```python
from build123d import *

# Parameters (mm, degrees)
SKETCH1_W               = 269.4
SKETCH1_H               = 265.6
BOSS_EXTRUDE1_DEPTH     = 3.175
CUT_EXTRUDE3_DEPTH      = 190.262390612
BOSS_EXTRUDE3_DEPTH     = 6.35
F_1_4_CLEARANCE_HOLE1_D = 6.7564
MIRROR2_COPY_1_DEPTH    = 6.35
MIRROR2_COPY_2_D        = 6.7564
CUT_EXTRUDE2_REACH      = 191.262
SKETCH15_W              = 0.944
SKETCH15_H              = 50.8
LPATTERN1_COUNT         = 8
LPATTERN1_PITCH         = 10
MIRROR3_COPY_1_REACH    = 191.262
MIRROR3_COPY_1_SKETCH_W = 0.944
MIRROR3_COPY_1_SKETCH_H = 50.8
MIRROR3_COPY_2_REACH    = 191.262
MIRROR3_COPY_2_SKETCH_W = 0.944
MIRROR3_COPY_2_SKETCH_H = 50.8
MIRROR3_COPY_3_REACH    = 191.262
MIRROR3_COPY_3_SKETCH_W = 0.944
MIRROR3_COPY_3_SKETCH_H = 50.8
MIRROR3_COPY_4_REACH    = 191.262
MIRROR3_COPY_4_SKETCH_W = 0.944
MIRROR3_COPY_4_SKETCH_H = 50.8
MIRROR3_COPY_5_REACH    = 191.262
MIRROR3_COPY_5_SKETCH_W = 0.944
MIRROR3_COPY_5_SKETCH_H = 50.8
MIRROR3_COPY_6_REACH    = 191.262
MIRROR3_COPY_6_SKETCH_W = 0.944
MIRROR3_COPY_6_SKETCH_H = 50.8
MIRROR3_COPY_7_REACH    = 191.262
MIRROR3_COPY_7_SKETCH_W = 0.944
MIRROR3_COPY_7_SKETCH_H = 50.8


with BuildPart() as part:
    # Sketch1 → Boss-Extrude1 (new, symmetric)
    with BuildSketch(Plane(origin=(0, 0, 0), x_dir=(1, 0, 0), z_dir=(0, 1, 0))):
        Rectangle(SKETCH1_W, SKETCH1_H)
    extrude(amount=BOSS_EXTRUDE1_DEPTH, both=True)

    # Sketch16 → Cut-Extrude3 (cut, through all)
    with BuildSketch(Plane(origin=(0, 3.175, 0), x_dir=(1, 0, 0), z_dir=(0, 1, 0))):
        Polygon((-134.7, 132.8), (-134.7, 91.434816919), (-99.990490133, 132.8), align=None)
        Polygon((99.990490133, 132.8), (134.7, 132.8), (134.7, 91.434816919), align=None)
        Polygon((134.7, -132.8), (134.7, -91.434816919), (99.990490133, -132.8), align=None)
        Polygon((-99.990490133, -132.8), (-134.7, -132.8), (-134.7, -91.434816919), align=None)
    extrude(amount=-CUT_EXTRUDE3_DEPTH, mode=Mode.SUBTRACT)

    # Sketch7 → Boss-Extrude3 (add)
    with BuildSketch(Plane(origin=(0, -3.175, 0), x_dir=(1, 0, 0), z_dir=(0, 1, 0))):
        Polygon((126.560486405, 125.832227239), (132.451914797, 118.811096288), (126.182387654, 101.585712032), (108.508102479, 122.649104887), align=None)
    boss_extrude3 = extrude(amount=BOSS_EXTRUDE3_DEPTH)

    # 1/4 Clearance Hole1 (through all)
    with Locations(Plane.XZ.offset(3.175)):
        with Locations((123.415994069, -117.211371709), (126.7498, -40), (0, -124.8498)):
            f_1_4_clearance_hole1 = Hole(F_1_4_CLEARANCE_HOLE1_D / 2)

    # Mirror1: Boss-Extrude3, 1/4 Clearance Hole1 across plane
    add(boss_extrude3.mirror(Plane.XY))
    add(f_1_4_clearance_hole1.mirror(Plane.XY), mode=Mode.SUBTRACT)

    # Mirror2: Boss-Extrude3, 1/4 Clearance Hole1 across plane
    add(boss_extrude3.mirror(Plane(origin=(0, 0, 0), x_dir=(0, 0, 1), z_dir=(1, 0, 0))))
    add(f_1_4_clearance_hole1.mirror(Plane(origin=(0, 0, 0), x_dir=(0, 0, 1), z_dir=(1, 0, 0))), mode=Mode.SUBTRACT)

    # Mirror2 copy 1 sketch → Mirror2 copy 1 (add)
    with BuildSketch(Plane(origin=(0, -3.175, 0), x_dir=(-1, 0, 0), z_dir=(0, 1, 0))):
        Polygon((126.560486405, 125.832227239), (132.451914797, 118.811096288), (126.182387654, 101.585712032), (108.508102479, 122.649104887), align=None)
    extrude(amount=MIRROR2_COPY_1_DEPTH)

    # Mirror2 copy 2 (through all)
    with Locations(Plane(origin=(0, -3.175, 0), x_dir=(-1, 0, 0), z_dir=(0, -1, 0))):
        with Locations((123.415994069, -117.211371709), (126.7498, -40), (0, -124.8498)):
            Hole(MIRROR2_COPY_2_D / 2)

    # Sketch15 → Cut-Extrude2 (cut, up to next)
    with BuildSketch(Plane(origin=(0, 3.175, 0), x_dir=(1, 0, 0), z_dir=(0, 1, 0)), mode=Mode.PRIVATE) as cut_extrude2_sk1:
        with Locations((-88.499, -97.4)):
            Rectangle(SKETCH15_W, SKETCH15_H)
    cut_extrude2_tool1 = extrude(cut_extrude2_sk1.sketch, amount=-CUT_EXTRUDE2_REACH, mode=Mode.PRIVATE) & part.part
    cut_extrude2 = cut_extrude2_tool1.solids().sort_by_distance((-88.499, 3.175, 97.4))[0]
    add(cut_extrude2, mode=Mode.SUBTRACT)

    # LPattern1: Cut-Extrude2 ×8
    with Locations(*[(i * LPATTERN1_PITCH, 0, 0) for i in range(1, LPATTERN1_COUNT)]):
        add(cut_extrude2, mode=Mode.SUBTRACT)

    # Mirror3: Cut-Extrude2 across plane
    add(cut_extrude2.mirror(Plane(origin=(0, 0, 0), x_dir=(0, 0, 1), z_dir=(1, 0, 0))), mode=Mode.SUBTRACT)

    # Mirror3 copy 1 sketch → Mirror3 copy 1 (cut, up to next)
    with BuildSketch(Plane(origin=(-10, 3.175, 0), x_dir=(-1, 0, 0), z_dir=(0, 1, 0)), mode=Mode.PRIVATE) as mirror3_copy_1_sk1:
        with Locations((-88.499, 97.4)):
            Rectangle(MIRROR3_COPY_1_SKETCH_W, MIRROR3_COPY_1_SKETCH_H)
    mirror3_copy_1_tool1 = extrude(mirror3_copy_1_sk1.sketch, amount=-MIRROR3_COPY_1_REACH, mode=Mode.PRIVATE) & part.part
    add(mirror3_copy_1_tool1.solids().sort_by_distance((78.499, 3.175, 97.4))[0], mode=Mode.SUBTRACT)

    # Mirror3 copy 2 sketch → Mirror3 copy 2 (cut, up to next)
    with BuildSketch(Plane(origin=(-20, 3.175, 0), x_dir=(-1, 0, 0), z_dir=(0, 1, 0)), mode=Mode.PRIVATE) as mirror3_copy_2_sk1:
        with Locations((-88.499, 97.4)):
            Rectangle(MIRROR3_COPY_2_SKETCH_W, MIRROR3_COPY_2_SKETCH_H)
    mirror3_copy_2_tool1 = extrude(mirror3_copy_2_sk1.sketch, amount=-MIRROR3_COPY_2_REACH, mode=Mode.PRIVATE) & part.part
    add(mirror3_copy_2_tool1.solids().sort_by_distance((68.499, 3.175, 97.4))[0], mode=Mode.SUBTRACT)

    # Mirror3 copy 3 sketch → Mirror3 copy 3 (cut, up to next)
    with BuildSketch(Plane(origin=(-30, 3.175, 0), x_dir=(-1, 0, 0), z_dir=(0, 1, 0)), mode=Mode.PRIVATE) as mirror3_copy_3_sk1:
        with Locations((-88.499, 97.4)):
            Rectangle(MIRROR3_COPY_3_SKETCH_W, MIRROR3_COPY_3_SKETCH_H)
    mirror3_copy_3_tool1 = extrude(mirror3_copy_3_sk1.sketch, amount=-MIRROR3_COPY_3_REACH, mode=Mode.PRIVATE) & part.part
    add(mirror3_copy_3_tool1.solids().sort_by_distance((58.499, 3.175, 97.4))[0], mode=Mode.SUBTRACT)

    # Mirror3 copy 4 sketch → Mirror3 copy 4 (cut, up to next)
    with BuildSketch(Plane(origin=(-40, 3.175, 0), x_dir=(-1, 0, 0), z_dir=(0, 1, 0)), mode=Mode.PRIVATE) as mirror3_copy_4_sk1:
        with Locations((-88.499, 97.4)):
            Rectangle(MIRROR3_COPY_4_SKETCH_W, MIRROR3_COPY_4_SKETCH_H)
    mirror3_copy_4_tool1 = extrude(mirror3_copy_4_sk1.sketch, amount=-MIRROR3_COPY_4_REACH, mode=Mode.PRIVATE) & part.part
    add(mirror3_copy_4_tool1.solids().sort_by_distance((48.499, 3.175, 97.4))[0], mode=Mode.SUBTRACT)

    # Mirror3 copy 5 sketch → Mirror3 copy 5 (cut, up to next)
    with BuildSketch(Plane(origin=(-50, 3.175, 0), x_dir=(-1, 0, 0), z_dir=(0, 1, 0)), mode=Mode.PRIVATE) as mirror3_copy_5_sk1:
        with Locations((-88.499, 97.4)):
            Rectangle(MIRROR3_COPY_5_SKETCH_W, MIRROR3_COPY_5_SKETCH_H)
    mirror3_copy_5_tool1 = extrude(mirror3_copy_5_sk1.sketch, amount=-MIRROR3_COPY_5_REACH, mode=Mode.PRIVATE) & part.part
    add(mirror3_copy_5_tool1.solids().sort_by_distance((38.499, 3.175, 97.4))[0], mode=Mode.SUBTRACT)

    # Mirror3 copy 6 sketch → Mirror3 copy 6 (cut, up to next)
    with BuildSketch(Plane(origin=(-60, 3.175, 0), x_dir=(-1, 0, 0), z_dir=(0, 1, 0)), mode=Mode.PRIVATE) as mirror3_copy_6_sk1:
        with Locations((-88.499, 97.4)):
            Rectangle(MIRROR3_COPY_6_SKETCH_W, MIRROR3_COPY_6_SKETCH_H)
    mirror3_copy_6_tool1 = extrude(mirror3_copy_6_sk1.sketch, amount=-MIRROR3_COPY_6_REACH, mode=Mode.PRIVATE) & part.part
    add(mirror3_copy_6_tool1.solids().sort_by_distance((28.499, 3.175, 97.4))[0], mode=Mode.SUBTRACT)

    # Mirror3 copy 7 sketch → Mirror3 copy 7 (cut, up to next)
    with BuildSketch(Plane(origin=(-70, 3.175, 0), x_dir=(-1, 0, 0), z_dir=(0, 1, 0)), mode=Mode.PRIVATE) as mirror3_copy_7_sk1:
        with Locations((-88.499, 97.4)):
            Rectangle(MIRROR3_COPY_7_SKETCH_W, MIRROR3_COPY_7_SKETCH_H)
    mirror3_copy_7_tool1 = extrude(mirror3_copy_7_sk1.sketch, amount=-MIRROR3_COPY_7_REACH, mode=Mode.PRIVATE) & part.part
    add(mirror3_copy_7_tool1.solids().sort_by_distance((18.499, 3.175, 97.4))[0], mode=Mode.SUBTRACT)


solid = part.part
```
Geometry check sheet. Reference: the model listing, model coordinates, mm. A direction names the side the tool comes from. Coordinates: 2 decimals unless noted, no trailing zeros. Order: outer loops, then holes, each group sorted by start corner. A loop starts at its lowest first (then second) coordinate and runs counter-clockwise, first axis right, second up. Notation, with made-up numbers: (79.25, 28.25) - (116.25, 28.25) arc R15 cw to (116.25, 39.25) - close; hole circle Ø8 at (9.25, 67.5). An arc over 180 degrees is marked (long way). Answer as a JSON object with one key per item and string values. Group by question number.
Item 1: Scan lines: probe 1 along Z at (x, y) = (0, 0); probe 2 along X at (y, z) = (0, -120); probe 3 along X at (y, z) = (0.5, 43). Record each from-to range of solid material in increasing order.
Item 2: Sectioned sample at C-C, the plane z = 86. Give the number of separate pieces and of enclosed holes in the cut face, and give its area (3 significant figures).
Item 3: Sectioned sample at A-A, the plane z = 40. Record the cut outline in (x, y) (3 decimals).
Item 4: Draft check along X on faces 1 (the face through (134.7, 0, 1)), 2 (the face through (-129.36, -0.04, 110.32)), 3 (the face through (-38.971, 0, 98)). Enter one of: +X half, -X half, draft (parallel to the pull), parting line (faces both ways), or undercut.
Item 5: Depth check by flat-ended pin: pin 1 Ø3 at (y, z) = (-0.5, 95) entering from -X; pin 2 Ø1.9 at (y, z) = (-0.5, 99.5) entering from -X. Enter the tip coordinate at first touch or a pass-through.
Item 6: Tool access check on faces 4 (the face through (130.5, 0.04, 96.44)), 5 (the face through (58.027, 0, 97)), 6 (the face through (-129.465, -0.044, 122.371)), 7 (the face through (104.31, 0.04, -127.65)). Record the directions out of +Z, -Z, +X, -X, +Y, -Y that give a thin tool (end or side, any length) a straight path to the whole face; none if there is none.
Item 7: Sectioned sample at B-B, the plane x = 0. Record the cut outline in (y, z) (3 decimals), and give its area (3 significant figures).
Resolved:
{
 "1": {"probe 1": "-132.8 to -128.23, -121.47 to 121.47, 128.23 to 132.8", "probe 2": "-131.45 to -125.32, -121.51 to 121.51, 125.32 to 131.45", "probe 3": "-134.7 to -128.3, -125.2 to 125.2, 128.3 to 134.7"},
 "2": {"separate pieces": "17", "enclosed holes": "0", "area": "1,610 mm^2"},
 "3": {"outline": "(-134.7, -3.175) - (-130.128, -3.175) - (-130.128, 3.175) - (-134.7, 3.175) - close; (-123.372, -3.175) - (123.372, -3.175) - (123.372, 3.175) - (-123.372, 3.175) - close; (130.128, -3.175) - (134.7, -3.175) - (134.7, 3.175) - (130.128, 3.175) - close"},
 "4": {"face 1": "+X half", "face 2": "-X half", "face 3": "undercut"},
 "5": {"pin 1": "x = -132.97", "pin 2": "x = -128.73"},
 "6": {"face 4": "+X, +Y, -Y", "face 5": "+Y, -Y", "face 6": "+Z, -X, +Y, -Y", "face 7": "-Z, +Y, -Y"},
 "7": {"outline": "(-3.175, -132.8) - (3.175, -132.8) - (3.175, -128.228) - (-3.175, -128.228) - close; (-3.175, -121.472) - (3.175, -121.472) - (3.175, 121.472) - (-3.175, 121.472) - close; (-3.175, 128.228) - (3.175, 128.228) - (3.175, 132.8) - (-3.175, 132.8) - close", "area": "1,600 mm^2"}
}
